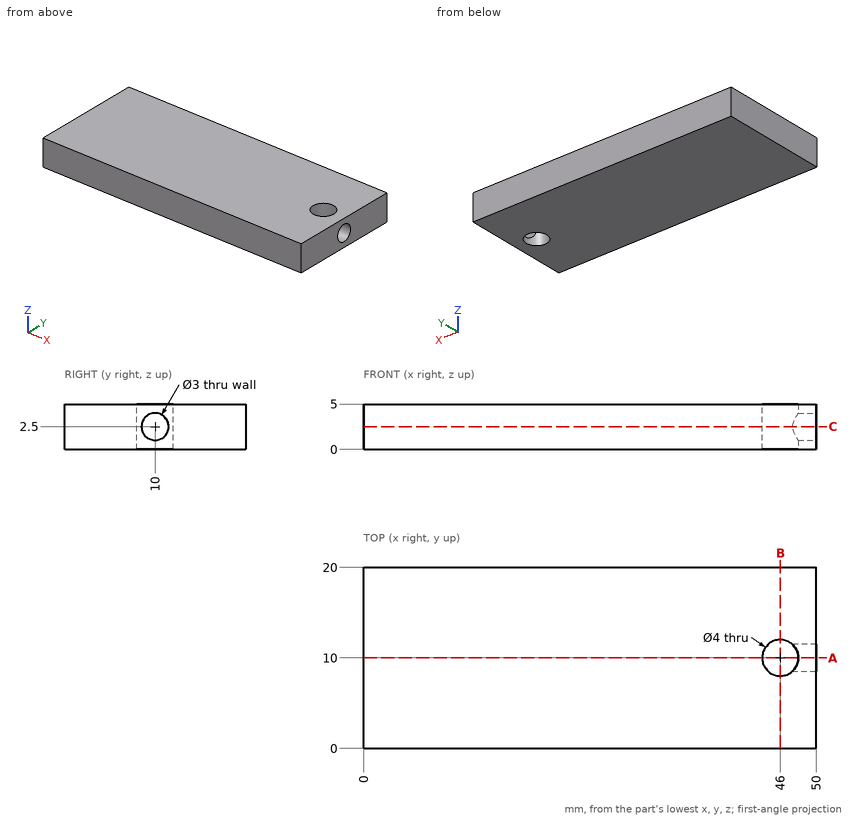
Part print with two shaded views. Sizes in mm from the minimum x, y, z corner. Give positions to 0.01 mm unless a question says otherwise; leave off trailing zeros. Order: outer loops, then holes, each group sorted by start corner. A loop starts at its lowest first (then second) coordinate and runs counter-clockwise, first axis right, second up.
(1) Saw through at A-A, the plane y = 10. Give the cut face in (x, z).
(2) Saw through at B-B, the plane x = 46. Give the cut face in (y, z), then the cut area to 3 significant figures.
(3) Flat gauge pin, fed straight in: pin 1 (2.5 mm diameter, centred on x = 46, y = 10, fed in from +Z). Where does the tip first touch, or does it go through?
(4) Drill centre lines: L1, parallel to Z at x = 49.2, y = 10; L2, parallel to Y at x = 46, z = 3.85; L3, parallel to X at y = 9, z = 3.95. Where is each one in solid material? Low to high.
(5) Saw through at C-C, the plane z = 2.5. Give the cut face in (x, y), then the cut area to 3 significant figures.
Results found:
1. outline: (0, 0) - (44, 0) - (44, 5) - (0, 5) - close; (48, 0) - (50, 0) - (50, 1) - (48, 1) - close; (48, 4) - (50, 4) - (50, 5) - (48, 5) - close
2. outline: (0, 0) - (8, 0) - (8, 5) - (0, 5) - close; (12, 0) - (20, 0) - (20, 5) - (12, 5) - close
2. area: 80.0 mm2
3. pin 1: passes through
4. L1: z = 0 to 1, 4 to 5
4. L2: y = 0 to 8, 12 to 20
4. L3: x = 0 to 44.27, 47.73 to 50
5. outline: (0, 0) - (50, 0) - (50, 8.5) - (47.32, 8.5) arc R2 cw (long way) to (47.32, 11.5) - (50, 11.5) - (50, 20) - (0, 20) - close
5. area: 981 mm2
